from build123d import *

# Parameters (mm, degrees)
SKETCH2_R           = 12.5
SKETCH2_R_2         = 7.5
BOSS_EXTRUDE1_DEPTH = 6
SKETCH3_R           = 10.5
CUT_EXTRUDE1_DEPTH  = 3
SKETCH4_R           = 3.05
CUT_EXTRUDE2_DEPTH  = 11
SKETCH5_R           = 2.2
CUT_EXTRUDE3_DEPTH  = 11
SKETCH6_R           = 57
SKETCH6_R_2         = 54
CUT_EXTRUDE4_DEPTH  = 2


with BuildPart() as part:
    # Sketch1 → Revolve1 (revolve)
    with BuildSketch(Plane.XY):
        Polygon((0, 0), (-67.5, 0), (-67.5, -5), (-50, -5), (-50, -10), (0, -10), align=None)
    revolve(axis=Axis((0, -10, 0), (0, 1, 0)))

    # Sketch2 → Boss-Extrude1 (add)
    with BuildSketch(Plane(origin=(0, 0, 0), x_dir=(1, 0, 0), z_dir=(0, 1, 0))):
        with Locations((0, -4)):
            Circle(SKETCH2_R)
        with Locations((0, -4)):
            Circle(SKETCH2_R_2, mode=Mode.SUBTRACT)
    extrude(amount=BOSS_EXTRUDE1_DEPTH)

    # Sketch3 → Cut-Extrude1 (cut)
    with BuildSketch(Plane.XZ.offset(10)):
        with Locations((0, 4)):
            Circle(SKETCH3_R)
    extrude(amount=-CUT_EXTRUDE1_DEPTH, mode=Mode.SUBTRACT)

    # Sketch4 → Cut-Extrude2 (cut, through all)
    with BuildSketch(Plane(origin=(0, 0, 0), x_dir=(1, 0, 0), z_dir=(0, 1, 0))):
        with Locations((0, -4)):
            Circle(SKETCH4_R)
    extrude(amount=-CUT_EXTRUDE2_DEPTH, mode=Mode.SUBTRACT)

    # Sketch5 → Cut-Extrude3 (cut, through all)
    with BuildSketch(Plane(origin=(0, 0, 0), x_dir=(1, 0, 0), z_dir=(0, 1, 0))):
        with Locations((0, 62)):
            Circle(SKETCH5_R)
        with Locations((62, 0)):
            Circle(SKETCH5_R)
        with Locations((0, -62)):
            Circle(SKETCH5_R)
        with Locations((-62, 0)):
            Circle(SKETCH5_R)
    extrude(amount=-CUT_EXTRUDE3_DEPTH, mode=Mode.SUBTRACT)

    # Sketch6 → Cut-Extrude4 (cut)
    with BuildSketch(Plane.XZ.offset(5)):
        Circle(SKETCH6_R)
        Circle(SKETCH6_R_2, mode=Mode.SUBTRACT)
    extrude(amount=-CUT_EXTRUDE4_DEPTH, mode=Mode.SUBTRACT)


solid = part.part
Input: part model. Units: mm. Frame: model coordinates. A direction names the side the tool comes from. Round coordinates to 2 decimals unless told otherwise and drop trailing zeros. Order: outer loops, then holes, each group sorted by start corner. A loop starts at its lowest first (then second) coordinate and runs counter-clockwise, first axis right, second up.
1. Material intervals for line 1 (Z direction, x = 46.5, y = -4.75); line 2 (X direction, y = 2.4, z = 4); line 3 (Z direction, x = 0, y = -9.15), sorted ascending.
The answers:
line 1: z = -48.93 to -32.97, -27.45 to 27.45, 32.97 to 48.93
line 2: x = -12.5 to -7.5, 7.5 to 12.5
line 3: z = -50 to -6.5, 14.5 to 50
2. Cut plane C-C, the plane z = -11. Output: boundary loops of the cut face in (x, y) (3 decimals), then the cut area to 3 significant figures.
The answers:
outline: (-66.598, -5) - (-55.929, -5) - (-55.929, -3) - (-52.868, -3) - (-52.868, -5) - (-48.775, -5) - (-48.775, -10) - (48.775, -10) - (48.775, -5) - (52.868, -5) - (52.868, -3) - (55.929, -3) - (55.929, -5) - (66.598, -5) - (66.598, 0) - (-66.598, 0) - close
area: 1,140 mm2
3. Set-up query: faces 4 (the face through (-48, -5, -16)), 5 (the face through (-0.477, -2.465, -59.852)), 6 (the face through (-5.5, 3, -1.1)). Return all of +Z, -Z, +X, -X, +Y, -Y with unobstructed straight access to the full face (end or side cutting, diameter ignored); none if empty.
The answers:
face 4: -Y
face 5: +Y, -Y
face 6: +Y
4. Pin query (flat end, axial travel): P1, Ø6.5, axis at x = 1, z = 5, coming from the -Y side; P2, Ø10, axis at x = 25, z = -26.5, coming from the +Y side; P3, Ø5.5, axis at x = 62, z = 0, coming from the -Y side; P4, Ø12, axis at x = 3.5, z = 2.5, coming from the +Y side. Return the tip coordinate at first contact, or that it passes through.
The answers:
P1: stops at y = -7
P2: stops at y = 0
P3: stops at y = -5
P4: stops at y = 6
5. Cut plane B-B, the plane x = 62. Output: boundary loops of the cut face in (y, z), then the cut area to 3 significant figures.
The answers:
outline: (-5, -26.69) - (0, -26.69) - (0, -2.2) - (-5, -2.2) - close; (-5, 2.2) - (0, 2.2) - (0, 26.69) - (-5, 26.69) - close
area: 245 mm2
6. Mould query, pull axis X, two halves, no side actions, for faces 1 (the face through (-0.1, 0, 0.8)), 2 (the face through (1, -10, -10)), 3 (the face through (-2.71, 2.958, 16.203)). Classes: released by +X, released by -X, zero draft, split by the parting line, or undercut.
The answers:
face 1: undercut
face 2: zero draft
face 3: split by the parting line
7. Cut plane D-D, the plane x = -44.5. Output: boundary loops of the cut face in (y, z).
The answers:
outline: (-10, -22.8) - (-5, -22.8) - (-5, -30.59) - (-3, -30.59) - (-3, -35.62) - (-5, -35.62) - (-5, -50.75) - (0, -50.75) - (0, 50.75) - (-5, 50.75) - (-5, 35.62) - (-3, 35.62) - (-3, 30.59) - (-5, 30.59) - (-5, 22.8) - (-10, 22.8) - close
